Could you check a few things on this model? Use its own coordinates, in mm. A direction names the side the tool comes from. Give positions to 0.01 mm unless a question says otherwise; leave off trailing zeros. Loops run counter-clockwise (first coordinate to the right, second up) from the corner with the lowest first, then second, coordinate; pieces in that order, holes last. Notation, with made-up numbers: M 3,-17 L 10,-17 A20 cw 10,-12 Z; hole C -30.75,-31 d9. An arc over 180 degrees is marked long. Use a Markdown table: item, result. Add a question column.
1) Which directions (+Z, -Z, +X, -X, +Y, -Y) give clear straight access to the entire face, cutting with the end or side of a thin tool? Please do faces 1 (the flat face through (4, 4, 9.398)), 2 (the flat face through (3, -8, 0)), 3 (the cylindrical face through (-2.75, -12.4, 11.03)).
2) If I drill on line 1 along Y through (x, z) = (0, 7.65); line 2 along Y through (x, z) = (0, 11.6); line 3 along Z through (x, y) = (-1.5, -16), over which ranges is the centre line in solid material (lowest first)? Write a range as [from, to].
3) We'd pull the mould along X, two halves only. Please class faces 4 (the cylindrical face through (-6.117, 1.926, 7.08)), 5 (the flat face through (-12, 8, 9.398)), 6 (the cylindrical face through (-2.75, -12.4, 1.63)): +X half, -X half, draft (parallel to the pull), parting line (faces both ways), or undercut.
4) Suppose I cut it at D-D on x = -12. List the corners of the cut face in (y, z) for me.
5) Suppose I cut it at C-C on z = 10. List the corners of the cut face in (x, y) for me, and give its area (3 significant figures).
6) Will these pins go through, and if not, where does the flat tip stop? pin 1 Ø2 at (x, z) = (-4.5, 3.5) entering from +Y; pin 2 Ø8.5 at (x, y) = (0.5, -3) entering from -Z; pin 3 Ø6.5 at (x, y) = (2, 1.5) entering from -Z.
7) Suppose I cut it at A-A on x = 0. List the corners of the cut face in (y, z) for me (1 decimal).
```python
from build123d import *

# Parameters (mm, degrees)
SKETCH1_R           = 12.7
BOSS_EXTRUDE1_DEPTH = 12.7
SKETCH2_R           = 17.78
BOSS_EXTRUDE2_DEPTH = 3.048
SKETCH5_R           = 6.4135
CUT_EXTRUDE1_DEPTH  = 9.398
SKETCH6_R           = 5.334
CUT_EXTRUDE2_DEPTH  = 29.169962726
SKETCH7_R           = 8.255
CUT_EXTRUDE3_DEPTH  = 4.826


with BuildPart() as part:
    # Sketch1 → Boss-Extrude1 (new body)
    with BuildSketch(Plane.XY):
        Circle(SKETCH1_R)
    extrude(amount=BOSS_EXTRUDE1_DEPTH)

    # Sketch2 → Boss-Extrude2 (add, symmetric)
    with BuildSketch(Plane.XY.offset(6.35)):
        with Locations(Location((0, 0, 0), (0, 0, 180))):
            Circle(SKETCH2_R)
    extrude(amount=BOSS_EXTRUDE2_DEPTH, both=True)

    # Sketch5 → Cut-Extrude1 (cut)
    with BuildSketch(Plane(origin=(0, 0, 0), x_dir=(-1, 0, 0), z_dir=(0, 0, -1))):
        Circle(SKETCH5_R)
    extrude(amount=-CUT_EXTRUDE1_DEPTH, mode=Mode.SUBTRACT)

    # Sketch6 → Cut-Extrude2 (cut, through all)
    with BuildSketch(Plane.XY.offset(12.7)):
        Circle(SKETCH6_R)
    extrude(amount=-CUT_EXTRUDE2_DEPTH, mode=Mode.SUBTRACT)

    # Sketch7 → Cut-Extrude3 (cut)
    with BuildSketch(Plane(origin=(0, 0, 0), x_dir=(-1, 0, 0), z_dir=(0, 0, -1))):
        Circle(SKETCH7_R)
    extrude(amount=-CUT_EXTRUDE3_DEPTH, mode=Mode.SUBTRACT)


solid = part.part
```
Answer block:
| question | item | result |
|---|---|---|
| 1 | face 1 | -Z |
| 1 | face 2 | -Z, +X, -X, +Y, -Y |
| 1 | face 3 | +Z |
| 2 | line 1 | y = [-17.78, -6.41], [6.41, 17.78] |
| 2 | line 2 | y = [-12.7, -5.33], [5.33, 12.7] |
| 2 | line 3 | z = [3.3, 9.4] |
| 3 | face 4 | undercut |
| 3 | face 5 | draft |
| 3 | face 6 | parting line |
| 4 | outline | M -13.12,3.3 L -4.16,3.3 L -4.16,0 L 4.16,0 L 4.16,3.3 L 13.12,3.3 L 13.12,9.4 L 4.16,9.4 L 4.16,12.7 L -4.16,12.7 L -4.16,9.4 L -13.12,9.4 Z |
| 5 | outline | C 0,0 d25.4; hole C 0,0 d10.67 |
| 5 | area | 417 mm^2 |
| 6 | pin 1 | stops at y = 17.43 |
| 6 | pin 2 | stops at z = 4.83 |
| 6 | pin 3 | stops at z = 9.4 |
| 7 | outline | M -17.8,3.3 L -12.7,3.3 L -12.7,0 L -8.3,0 L -8.3,4.8 L -6.4,4.8 L -6.4,9.4 L -5.3,9.4 L -5.3,12.7 L -12.7,12.7 L -12.7,9.4 L -17.8,9.4 Z; M 5.3,9.4 L 6.4,9.4 L 6.4,4.8 L 8.3,4.8 L 8.3,0 L 12.7,0 L 12.7,3.3 L 17.8,3.3 L 17.8,9.4 L 12.7,9.4 L 12.7,12.7 L 5.3,12.7 Z |
